Verification items for the finished model (mm, model axes). Face numbers are marked on the shaded views. A direction names the side the tool comes from. Coordinates: 2 decimals unless noted, no trailing zeros. Order: outer loops, then holes, each group sorted by start corner. A loop starts at its lowest first (then second) coordinate and runs counter-clockwise, first axis right, second up.
Q1. Thickness scan on line 1 (Z direction, x = -7.5, y = 0.4); line 2 (Z direction, x = -2.5, y = 10); line 3 (X direction, y = 1, z = 13). Record the ranges inside material, lowest first.
Q2. Depth check by flat-ended pin: P1, Ø3.5, axis at x = 7.5, z = 13, coming from the +Y side. Enter the tip coordinate at first touch or a pass-through.
Q3. Draft check along X on the marked faces 1, 2 and 3. Enter one of: pulls with the +X half, pulls with the -X half, needs draft (parallel to the pull), parting line crosses it, or undercut.
Q4. Set-up check for the marked faces 4 and 5: record each of +Z, -Z, +X, -X, +Y, -Y from which the full face is reachable in a straight line by a thin tool's end or side.
Q5. Cross-section at C-C, the plane x = 15.5. Record the boundary of the cut face in (y, z).
Q6. Cross-section at A-A, the plane z = -22. Record the boundary of the cut face in (x, y), and give its area (3 significant figures).
Q7. Cross-section at D-D, the plane y = 10.75. Record the boundary of the cut face in (x, z).
Q8. Cross-section at B-B, the plane x = -7.5. Record the boundary of the cut face in (y, z), and give its area (3 significant figures).
from build123d import *

# Parameters (mm, degrees)
SKETCH1_W           = 51.5
SKETCH1_H           = 65
SKETCH1_R           = 1.5025
BOSS_EXTRUDE1_DEPTH = 15
SKETCH2_W           = 49.5
SKETCH2_H           = 14
CUT_EXTRUDE1_DEPTH  = 13


with BuildPart() as part:
    # Sketch1 → Boss-Extrude1 (new body)
    with BuildSketch(Plane(origin=(0, 0, 0), x_dir=(1, 0, 0), z_dir=(0, 1, 0))):
        Rectangle(SKETCH1_W, SKETCH1_H)
        with Locations((-7.5, -13)):
            Circle(SKETCH1_R, mode=Mode.SUBTRACT)
        with Locations((7.5, -13)):
            Circle(SKETCH1_R, mode=Mode.SUBTRACT)
        with Locations((7.5, 22)):
            Circle(SKETCH1_R, mode=Mode.SUBTRACT)
        with Locations((-7.5, 22)):
            Circle(SKETCH1_R, mode=Mode.SUBTRACT)
    extrude(amount=BOSS_EXTRUDE1_DEPTH)

    # Sketch2 → Cut-Extrude1 (cut)
    with BuildSketch(Plane(origin=(0, 15, 0), x_dir=(1, 0, 0), z_dir=(0, 1, 0))):
        with Locations((0, -8.5)):
            Rectangle(SKETCH2_W, SKETCH2_H)
        with Locations((0, -24.5)):
            Rectangle(SKETCH2_W, SKETCH2_H)
        with Locations((0, 24.5)):
            Rectangle(SKETCH2_W, SKETCH2_H)
        with Locations((0, 8.5)):
            Rectangle(SKETCH2_W, SKETCH2_H)
    extrude(amount=-CUT_EXTRUDE1_DEPTH, mode=Mode.SUBTRACT)


solid = part.part
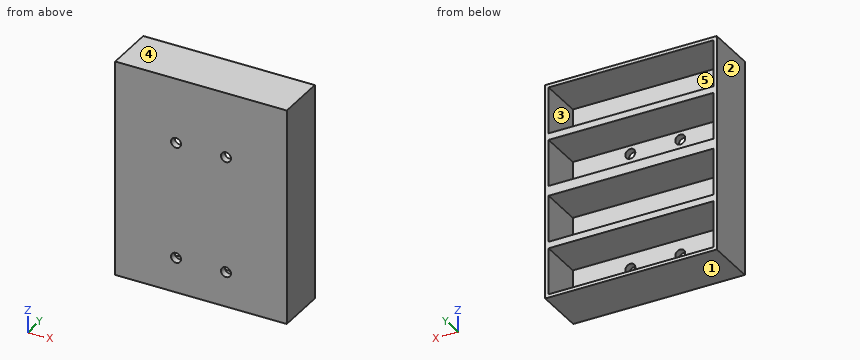
Check values:
1. line 1: z = -32.5 to -23.5, -20.5 to 11.5, 14.5 to 32.5
1. line 2: z = -32.5 to -31.5, -17.5 to -15.5, -1.5 to 1.5, 15.5 to 17.5, 31.5 to 32.5
1. line 3: x = -25.75 to -9, -6 to 6, 9 to 25.75
2. P1: stops at y = 2
3. face 1: needs draft
3. face 2: pulls with the -X half
3. face 3: undercut
4. face 4: +Z, +X, -X, +Y, -Y
4. face 5: +Y
5. outline: (0, -32.5) - (15, -32.5) - (15, -31.5) - (2, -31.5) - (2, -17.5) - (15, -17.5) - (15, -15.5) - (2, -15.5) - (2, -1.5) - (15, -1.5) - (15, 1.5) - (2, 1.5) - (2, 15.5) - (15, 15.5) - (15, 17.5) - (2, 17.5) - (2, 31.5) - (15, 31.5) - (15, 32.5) - (0, 32.5) - close
6. outline: (-25.75, 0) - (-9, 0) - (-9, 2) - (-24.75, 2) - (-24.75, 15) - (-25.75, 15) - close; (-6, 0) - (6, 0) - (6, 2) - (-6, 2) - close; (9, 0) - (25.75, 0) - (25.75, 15) - (24.75, 15) - (24.75, 2) - (9, 2) - close
6. area: 117 mm2
7. outline: (-25.75, -32.5) - (25.75, -32.5) - (25.75, 32.5) - (-25.75, 32.5) - close; hole (-24.75, -31.5) - (24.75, -31.5) - (24.75, -17.5) - (-24.75, -17.5) - close; hole (-24.75, -15.5) - (24.75, -15.5) - (24.75, -1.5) - (-24.75, -1.5) - close; hole (-24.75, 1.5) - (24.75, 1.5) - (24.75, 15.5) - (-24.75, 15.5) - close; hole (-24.75, 17.5) - (24.75, 17.5) - (24.75, 31.5) - (-24.75, 31.5) - close
8. outline: (0, -32.5) - (15, -32.5) - (15, -31.5) - (2, -31.5) - (2, -23.5) - (0, -23.5) - close; (0, -20.5) - (2, -20.5) - (2, -17.5) - (15, -17.5) - (15, -15.5) - (2, -15.5) - (2, -1.5) - (15, -1.5) - (15, 1.5) - (2, 1.5) - (2, 11.5) - (0, 11.5) - close; (0, 14.5) - (2, 14.5) - (2, 15.5) - (15, 15.5) - (15, 17.5) - (2, 17.5) - (2, 31.5) - (15, 31.5) - (15, 32.5) - (0, 32.5) - close
8. area: 235 mm2
